CAD build for the part. Positions are in the model's coordinates, mm. A direction names the side the tool comes from. Coordinates: 2 decimals unless noted, no trailing zeros. Answer as CSV lines item,"result". Start each with the question number.
```python
from build123d import *

# Parameters (mm, degrees)
SKETCH_1_R               = 30
EXTRUDE_1_DEPTH          = 8
FILLET_1_R               = 100
FILLET_3_R               = 100
EXTRUDE_2_DEPTH          = 10
FILLET_2_R               = 10
CHAMFER_1_SIZE           = 5
CUT_EXTRUDE_4_DEPTH      = 514.758413114
CUT_EXTRUDE_4_DEPTH_BACK = 514.758413114
SKETCH_7_R               = 4.3
CUT_EXTRUDE_5_DEPTH      = 514.758413114
CUT_EXTRUDE_5_DEPTH_BACK = 514.758413114
SKETCH_8_R               = 2.25
SKETCH_9_R               = 4
CUT_EXTRUDE_6_DEPTH      = 4.4
SKETCH_10_W              = 20
SKETCH_10_H              = 20
CUT_EXTRUDE_7_DEPTH      = 4
FILLET_4_R               = 3


with BuildPart() as part:
    # 草图1 → 凸台-拉伸1 (new body)
    with BuildSketch(Plane.XY):
        Polygon((0, 280), (861.751390409, 0), (0, 0), (-100, 0), (-961.751390409, 0), (-100, 280), align=None)
        with Locations((200, 100)):
            Circle(SKETCH_1_R, mode=Mode.SUBTRACT)
        with Locations(Location((-300, 100, 0), (0, 0, 180))):
            Circle(SKETCH_1_R, mode=Mode.SUBTRACT)
    extrude(amount=EXTRUDE_1_DEPTH)

    # 圆角1
    fillet_1_edges = [part.edges().sort_by_distance(p)[0] for p in [
        (861.751390409, 0, 4),
    ]]
    fillet(fillet_1_edges, radius=FILLET_1_R)

    # 圆角3
    fillet_3_edges = [part.edges().sort_by_distance(p)[0] for p in [
        (-961.751390409, 0, 4),
    ]]
    fillet(fillet_3_edges, radius=FILLET_3_R)

    # 草图2 → 凸台-拉伸2 (add)
    with BuildSketch(Plane.XY):
        with BuildLine():
            Line((0, 280), (-100, 280))
            Line((-100, 280), (-361.277938379, 195.10565163))
            ThreePointArc((-361.277938379, 195.10565163), (-429.145073001, 84.356553496), (-330.376238942, 0))
            Line((-330.376238942, 0), (230.376238942, 0))
            ThreePointArc((230.376238942, 0), (329.145073001, 84.356553496), (261.277938379, 195.10565163))
            Line((261.277938379, 195.10565163), (0, 280))
        make_face()
        Polygon((10, 266.236180795), (122.241374643, 229.766747442), (10, 35.358983849), align=None, mode=Mode.SUBTRACT)
        with BuildLine():
            Line((230.376238942, 10), (30, 10))
            Line((30, 10), (151.410485182, 220.289128906))
            Line((151.410485182, 220.289128906), (258.187768435, 185.595086467))
            ThreePointArc((258.187768435, 185.595086467), (319.268189595, 85.920898146), (230.376238942, 10))
        make_face(mode=Mode.SUBTRACT)
        Polygon((-110, 266.236180795), (-110, 35.358983849), (-222.241374643, 229.766747442), align=None, mode=Mode.SUBTRACT)
        with BuildLine():
            Line((-358.187768435, 185.595086467), (-251.410485182, 220.289128906))
            Line((-251.410485182, 220.289128906), (-130, 10))
            Line((-130, 10), (-330.376238942, 10))
            ThreePointArc((-330.376238942, 10), (-419.268189595, 85.920898146), (-358.187768435, 185.595086467))
        make_face(mode=Mode.SUBTRACT)
    extrude(amount=-EXTRUDE_2_DEPTH)

    # 圆角2
    fillet_2_edges = [part.edges().sort_by_distance(p)[0] for p in [
        (-110, 35.358983849, -5),
        (-110, 266.236180795, -5),
        (-130, 10, -5),
        (10, 266.236180795, -5),
        (10, 35.358983849, -5),
        (151.410485182, 220.289128906, -5),
        (30, 10, -5),
        (-251.410485182, 220.289128906, -5),
        (122.241374643, 229.766747442, -5),
        (-222.241374643, 229.766747442, -5),
    ]]
    fillet(fillet_2_edges, radius=FILLET_2_R)

    # 倒角1
    chamfer_1_edges = [part.edges().sort_by_distance(p)[0] for p in [
        (-230.63896919, 237.552825815, 8),
        (130.63896919, 237.552825815, 8),
        (329.145073001, 84.356553496, 8),
        (-50, 0, 8),
        (-429.145073001, 84.356553496, 8),
        (-230.63896919, 237.552825815, -10),
        (130.63896919, 237.552825815, -10),
        (329.145073001, 84.356553496, -10),
        (-50, 0, -10),
        (-429.145073001, 84.356553496, -10),
    ]]
    chamfer(chamfer_1_edges, length=CHAMFER_1_SIZE)

    # 草图7 → 切除-拉伸4 (cut, two sides: drawn at the far end of the back side and taken through both)
    with BuildSketch(Plane.XY.offset(8).offset(-CUT_EXTRUDE_4_DEPTH_BACK)):
        with Locations((20, 217)):
            Circle(SKETCH_7_R)
        with Locations((-10, 217)):
            Circle(SKETCH_7_R)
        with Locations((20, 177)):
            Circle(SKETCH_7_R)
        with Locations((-10, 177)):
            Circle(SKETCH_7_R)
        with Locations((20, 89)):
            Circle(SKETCH_7_R)
        with Locations((-10, 89)):
            Circle(SKETCH_7_R)
        with Locations((20, 49)):
            Circle(SKETCH_7_R)
        with Locations((-10, 49)):
            Circle(SKETCH_7_R)
        with Locations(Location((-90, 49, 0), (0, 0, 180))):
            Circle(SKETCH_7_R)
        with Locations(Location((-120, 49, 0), (0, 0, 180))):
            Circle(SKETCH_7_R)
        with Locations(Location((-90, 89, 0), (0, 0, 180))):
            Circle(SKETCH_7_R)
        with Locations(Location((-120, 89, 0), (0, 0, 180))):
            Circle(SKETCH_7_R)
        with Locations(Location((-90, 177, 0), (0, 0, 180))):
            Circle(SKETCH_7_R)
        with Locations(Location((-120, 177, 0), (0, 0, 180))):
            Circle(SKETCH_7_R)
        with Locations(Location((-90, 217, 0), (0, 0, 180))):
            Circle(SKETCH_7_R)
        with Locations(Location((-120, 217, 0), (0, 0, 180))):
            Circle(SKETCH_7_R)
    extrude(amount=CUT_EXTRUDE_4_DEPTH + CUT_EXTRUDE_4_DEPTH_BACK, mode=Mode.SUBTRACT)

    # 草图8 → 切除-拉伸5 (cut, two sides: drawn at the far end of the back side and taken through both)
    with BuildSketch(Plane.XY.offset(8).offset(-CUT_EXTRUDE_5_DEPTH_BACK)):
        with Locations((200, 141.5)):
            Circle(SKETCH_8_R)
        with Locations((229.344931419, 129.344931419)):
            Circle(SKETCH_8_R)
        with Locations((241.5, 100)):
            Circle(SKETCH_8_R)
        with Locations((229.344931419, 70.655068581)):
            Circle(SKETCH_8_R)
        with Locations((200, 58.5)):
            Circle(SKETCH_8_R)
        with Locations((170.655068581, 70.655068581)):
            Circle(SKETCH_8_R)
        with Locations((158.5, 100)):
            Circle(SKETCH_8_R)
        with Locations((170.655068581, 129.344931419)):
            Circle(SKETCH_8_R)
        with Locations((-270.655068581, 129.344931419)):
            Circle(SKETCH_8_R)
        with Locations((-258.5, 100)):
            Circle(SKETCH_8_R)
        with Locations((-270.655068581, 70.655068581)):
            Circle(SKETCH_8_R)
        with Locations((-300, 58.5)):
            Circle(SKETCH_8_R)
        with Locations((-329.344931419, 70.655068581)):
            Circle(SKETCH_8_R)
        with Locations((-341.5, 100)):
            Circle(SKETCH_8_R)
        with Locations((-329.344931419, 129.344931419)):
            Circle(SKETCH_8_R)
        with Locations((-300, 141.5)):
            Circle(SKETCH_8_R)
    extrude(amount=CUT_EXTRUDE_5_DEPTH + CUT_EXTRUDE_5_DEPTH_BACK, mode=Mode.SUBTRACT)

    # 草图9 → 切除-拉伸6 (cut)
    with BuildSketch(Plane.XY.offset(8)):
        with Locations((-300, 141.5)):
            Circle(SKETCH_9_R)
        with Locations((-270.655068581, 129.344931419)):
            Circle(SKETCH_9_R)
        with Locations((-258.5, 100)):
            Circle(SKETCH_9_R)
        with Locations((-270.655068581, 70.655068581)):
            Circle(SKETCH_9_R)
        with Locations((-300, 58.5)):
            Circle(SKETCH_9_R)
        with Locations((-329.344931419, 70.655068581)):
            Circle(SKETCH_9_R)
        with Locations((-341.5, 100)):
            Circle(SKETCH_9_R)
        with Locations((-329.344931419, 129.344931419)):
            Circle(SKETCH_9_R)
        with Locations(Location((229.344931419, 129.344931419, 0), (0, 0, 180))):
            Circle(SKETCH_9_R)
        with Locations(Location((241.5, 100, 0), (0, 0, 180))):
            Circle(SKETCH_9_R)
        with Locations(Location((229.344931419, 70.655068581, 0), (0, 0, 180))):
            Circle(SKETCH_9_R)
        with Locations(Location((200, 58.5, 0), (0, 0, 180))):
            Circle(SKETCH_9_R)
        with Locations(Location((170.655068581, 70.655068581, 0), (0, 0, 180))):
            Circle(SKETCH_9_R)
        with Locations(Location((158.5, 100, 0), (0, 0, 180))):
            Circle(SKETCH_9_R)
        with Locations(Location((170.655068581, 129.344931419, 0), (0, 0, 180))):
            Circle(SKETCH_9_R)
        with Locations(Location((200, 141.5, 0), (0, 0, 180))):
            Circle(SKETCH_9_R)
    extrude(amount=-CUT_EXTRUDE_6_DEPTH, mode=Mode.SUBTRACT)

    # 草图10 → 切除-拉伸7 (cut)
    with BuildSketch(Plane(origin=(0, 0, -10), x_dir=(-1, 0, 0), z_dir=(0, 0, -1))):
        with Locations((50, 100)):
            Rectangle(SKETCH_10_W, SKETCH_10_H)
    extrude(amount=-CUT_EXTRUDE_7_DEPTH, mode=Mode.SUBTRACT)

    # 圆角4
    fillet_4_edges = [part.edges().sort_by_distance(p)[0] for p in [
        (-40, 90, -8),
        (-40, 110, -8),
        (-60, 110, -8),
        (-60, 90, -8),
    ]]
    fillet(fillet_4_edges, radius=FILLET_4_R)


solid = part.part
```
1. Tool access for faces 5 (the face through (-328.615, 90.989, 3.944)), 6 (the face through (-309.343, 201.466, -4.93)): list every direction of +Z, -Z, +X, -X, +Y, -Y with a clear straight run to the whole face (end or side of a thin tool).
2. Wall check: line 1 (Y direction, x = -90, z = 1.75); line 2 (Y direction, x = -177.5, z = -6.5); line 3 (X direction, y = 180.5, z = 4.5). Give the ranges that are in metal, low to high.
3. Flat gauge pins, fed straight in: P1, Ø3, axis at x = -323, z = -7.5, coming from the +Y side; P2, Ø1, axis at x = -317, z = -7.5, coming from the -Y side; P3, Ø3, axis at x = -15.5, z = -7.5, coming from the -Y side; P4, Ø9, axis at x = 230, y = 72, coming from the +Z side. Where does each tip first touch, or does it go through?
4. Mould opens along Y. For faces 1 (the face through (-224.469, 236.892, 5.535)), 2 (the face through (-418.97, 84.16, -4.93)), 3 (the face through (324.2, 83.23, -9.69)), 4 (the face through (-52, 133, -10)) say: pulls with the +Y half, pulls with the -Y half, needs draft (parallel to the pull), parting line crosses it, or undercut.
Geometry check:
1,face 5,"+Z, -Z"
1,face 6,"-Z"
2,line 1,"0 to 44.7, 53.3 to 84.7, 93.3 to 172.7, 181.3 to 212.7, 221.3 to 280"
2,line 2,"1.5 to 10, 92.27 to 152.27, 244.3 to 253.24"
2,line 3,"-387.14 to -122.5, -117.5 to -92.5, -87.5 to -12.5, -7.5 to 17.5, 22.5 to 287.14"
3,P1,"y = 206.57"
3,P2,"y = 2"
3,P3,"y = 1"
3,P4,"z = 8"
4,face 1,"pulls with the +Y half"
4,face 2,"undercut"
4,face 3,"parting line crosses it"
4,face 4,"needs draft"
